Verification items for the finished model (mm, model axes). A direction names the side the tool comes from. Give positions to 0.01 mm unless a question says otherwise; leave off trailing zeros. Order: outer loops, then holes, each group sorted by start corner. A loop starts at its lowest first (then second) coordinate and runs counter-clockwise, first axis right, second up. Notation, with made-up numbers: (86.5, 34.5) -> (108.5, 34.5) arc R4 ccw to (108.5, 38.5) -> close; hole circle Ø4 at (-2.5, -20). An arc over 180 degrees is marked (long way). Return JSON: item names as keys, results as strings. Group by question number.
(1) Cross-section at D-D on y = -5.75. Enter the section's corners in (x, z).
(2) Cross-section at C-C on z = 2.8. Enter the section's corners in (x, y), then the cut area to 3 significant figures.
(3) Release check for a two-part mould opening along X. For faces 1 (the face through (-37.795, -9, 2)), 2 (the face through (21, 0, 2)), 3 (the face through (7.365, -10, 2)), 4 (the face through (3.683, -16, 2)) record: pulls with the +X half, pulls with the -X half, needs draft (parallel to the pull), parting line crosses it, or undercut.
(4) Cross-section at A-A on x = -20. Enter the section's corners in (y, z).
(5) Tool access check on faces 5 (the face through (-9.411, -9, 2)), 6 (the face through (-3.45, -16, 2)), 7 (the face through (0, -4.816, 2)). Record the directions out of +Z, -Z, +X, -X, +Y, -Y that give a thin tool (end or side, any length) a straight path to the whole face; none if there is none.
(6) Depth check by flat-ended pin: pin 1 Ø1.2 at (x, z) = (1, 1) entering from -Y. Enter the tip coordinate at first touch or a pass-through.
(7) Thickness scan on line 1 along X through (y, z) = (-15, 0.5); line 2 along X through (y, z) = (-4.25, 2.9); line 3 along Y through (x, z) = (-12, 3.45). Record the ranges inside material, lowest first.
(8) Cross-section at B-B on y = -9.75. Enter the section's corners in (x, z), then the cut area to 3 significant figures.
from build123d import *

# Parameters (mm, degrees)
F0_W     = 3.4498951863
F0_H     = 2.832734026
F0_H_2   = 2.2661872208
F1_DEPTH = 4


with BuildPart() as f1:
    # F0 (on Top) → F1 (new body)
    with BuildSketch(Plane.XY):
        with Locations((-1.7249475932, -12.4640292488)):
            Rectangle(F0_W, F0_H)
        with Locations((-1.7249475932, -5.9487414546)):
            Rectangle(F0_W, F0_H_2)
        Polygon((18.1294977665, 0), (3.1160083599, 0), (3.1160083599, -4.8156478442), (0, -4.8156478442), (0, -7.081835065), (3.1160083599, -7.081835065), (3.6825551651, -11.0476622358), (0, -11.0476622358), (0, -13.8803962618), (3.6825551651, -13.8803962618), (3.6825551651, -18.6960436404), (37.9586368799, -18.6960436404), (37.9586368799, 0), (32.2931706905, 0), align=None)
        Polygon((7.3651084676, -3.682554001), (33.4262624383, -3.9658271708), (33.4262624383, -15.2967637405), (7.3651084676, -15.2967637405), align=None, mode=Mode.SUBTRACT)
        Polygon((-3.4498951863, -7.081835065), (-3.4498951863, -4.8156478442), (-3.4498951863, 0), (-6.85604522, 0), (-37.7952493727, 0), (-37.7952493727, -18.6960436404), (-3.4498951863, -18.6960436404), (-3.4498951863, -13.8803962618), (-3.4498951863, -11.0476622358), align=None)
        Polygon((-32.9698696733, -14.3438782543), (-33.5375629365, -4.4092708267), (-9.4106579199, -4.4092708267), (-9.4106579199, -14.3438782543), align=None, mode=Mode.SUBTRACT)
    extrude(amount=F1_DEPTH)


solid = f1.part
Verdict:
{
 "1": {"outline": "(-37.8, 0) -> (-33.46, 0) -> (-33.46, 4) -> (-37.8, 4) -> close; (-9.41, 0) -> (7.37, 0) -> (7.37, 4) -> (-9.41, 4) -> close; (33.43, 0) -> (37.96, 0) -> (37.96, 4) -> (33.43, 4) -> close"},
 "2": {"outline": "(-37.8, -18.7) -> (-3.45, -18.7) -> (-3.45, -13.88) -> (3.68, -13.88) -> (3.68, -18.7) -> (37.96, -18.7) -> (37.96, 0) -> (3.12, 0) -> (3.12, -4.82) -> (-3.45, -4.82) -> (-3.45, 0) -> (-37.8, 0) -> close; hole (-33.54, -4.41) -> (-32.97, -14.34) -> (-9.41, -14.34) -> (-9.41, -4.41) -> close; hole (-3.45, -11.05) -> (3.68, -11.05) -> (3.12, -7.08) -> (-3.45, -7.08) -> close; hole (7.37, -15.3) -> (33.43, -15.3) -> (33.43, -3.97) -> (7.37, -3.68) -> close", "area": "787 mm²"},
 "3": {"face 1": "pulls with the -X half", "face 2": "needs draft", "face 3": "undercut", "face 4": "undercut"},
 "4": {"outline": "(-18.7, 0) -> (-14.34, 0) -> (-14.34, 4) -> (-18.7, 4) -> close; (-4.41, 0) -> (0, 0) -> (0, 4) -> (-4.41, 4) -> close"},
 "5": {"face 5": "+Z, -Z", "face 6": "+Z, -Z, -Y", "face 7": "+Z, -Z, +Y"},
 "6": {"pin 1": "y = -13.88"},
 "7": {"line 1": "-37.8 to -3.45, 3.68 to 7.37, 33.43 to 37.96", "line 2": "-37.8 to -3.45, 3.12 to 7.37, 33.43 to 37.96", "line 3": "-18.7 to -14.34, -4.41 to 0"},
 "8": {"outline": "(-37.8, 0) -> (-33.23, 0) -> (-33.23, 4) -> (-37.8, 4) -> close; (-9.41, 0) -> (-3.45, 0) -> (-3.45, 4) -> (-9.41, 4) -> close; (3.5, 0) -> (7.37, 0) -> (7.37, 4) -> (3.5, 4) -> close; (33.43, 0) -> (37.96, 0) -> (37.96, 4) -> (33.43, 4) -> close", "area": "75.7 mm²"}
}
